```python
from build123d import *

# Parameters (mm, degrees)
F1_DEPTH = 25.4
F3_DEPTH = 25.4


with BuildPart() as f1:
    # F0 (on Top) → F1 (new body)
    with BuildSketch(Plane.XY):
        Polygon((41.092899, 0), (0, 0), (6.345855, -42.114921), align=None)
    extrude(amount=F1_DEPTH)

    # F2 (on face) → F3 (cut)
    with BuildSketch(Plane.XY.offset(25.4)):
        Polygon((18.505031, -9.646224), (17.724764, -4.467904), (12.850075, -2.554476), (8.755653, -5.819366), (9.535919, -10.997685), (14.410608, -12.911114), align=None)
    extrude(amount=-F3_DEPTH, mode=Mode.SUBTRACT)


solid = f1.part
```
Verification items for the finished model (mm, model axes). A direction names the side the tool comes from. Round coordinates to 2 decimals unless told otherwise and drop trailing zeros. Write each loop counter-clockwise with the first axis right and the second up, starting at its lowest first coordinate (ties: lowest second). Pieces come first, ordered by that corner, then holes. Notation, with made-up numbers: (9.25, 37) -> (68.25, 37) arc R36 cw to (68.25, 75) -> close; hole circle Ø8 at (32.5, 77.5). An arc over 180 degrees is marked (long way). Write each question's results on one line, items separated by ' | '. Start each with the question number.
1. Material ranges on probe 1 along Y at (x, z) = (13, 22); probe 2 along X at (y, z) = (-8, 23.5); probe 3 along Y at (x, z) = (14, 6.25), recorded low to high. Write a range as from..to.
2. Cross-section at C-C (x = 13.5). Enter the section's corners in (y, z), then the cut area to 3 significant figures.
3. Depth check by flat-ended pin: P1, Ø6, axis at y = -9, z = 19.5, coming from the -X side; P2, Ø3, axis at y = -20, z = 21.5, coming from the +X side; P3, Ø4, axis at y = -14.5, z = 5, coming from the +X side. Enter the tip coordinate at first touch or a pass-through.
4. Draft check along X on faces 1 (the flat face through (16, -16, 0)), 2 (the flat face through (9.14, -8.37, 12.88)), 3 (the flat face through (3.13, -20.76, 12.52)). Enter one of: +X half, -X half, draft (parallel to the pull), parting line (faces both ways), or undercut.
5. Cross-section at A-A (y = -5). Enter the section's corners in (x, z).
6. Set-up check for faces 4 (the flat face through (21, 0, 13)), 5 (the flat face through (11.94, -11.94, 12.88)): record each of +Z, -Z, +X, -X, +Y, -Y from which the full face is reachable in a straight line by a thin tool's end or side.
7. Cross-section at D-D (y = -29). Enter the section's corners in (x, z).
8. Cross-section at B-B (z = 7.75). Enter the section's corners in (x, y), then the cut area to 3 significant figures.
Solutions:
1) probe 1: y = -34.05..-12.36, -2.61..0 | probe 2: x = 1.21..9.08, 18.26..34.49 | probe 3: y = -32.84..-12.75, -3.01..0
2) outline: (-33.44, 0) -> (-12.55, 0) -> (-12.55, 25.4) -> (-33.44, 25.4) -> close; (-2.81, 0) -> (0, 0) -> (0, 25.4) -> (-2.81, 25.4) -> close | area: 602 mm2
3) P1: stops at x = 0.9 | P2: stops at x = 25.83 | P3: stops at x = 30.78
4) face 1: draft | face 2: undercut | face 3: -X half
5) outline: (0.75, 0) -> (9.78, 0) -> (9.78, 25.4) -> (0.75, 25.4) -> close; (17.8, 0) -> (36.97, 0) -> (36.97, 25.4) -> (17.8, 25.4) -> close
6) face 4: +Z, -Z, +X, -X, +Y | face 5: +Z, -Z
7) outline: (4.37, 0) -> (17.17, 0) -> (17.17, 25.4) -> (4.37, 25.4) -> close
8) outline: (0, 0) -> (6.35, -42.11) -> (41.09, 0) -> close; hole (8.76, -5.82) -> (9.54, -11) -> (14.41, -12.91) -> (18.51, -9.65) -> (17.72, -4.47) -> (12.85, -2.55) -> close | area: 794 mm2
